Design review of the part shown in the three views and the two pictorial views. Dimensions are in mm from the part's minimum x, y and z. Round coordinates to 2 decimals unless told otherwise and drop trailing zeros. Loops run counter-clockwise (first coordinate to the right, second up) from the corner with the lowest first, then second, coordinate; pieces in that order, holes last. Notation, with made-up numbers: M -29,48.25 L -6,48.25 A30 cw -6,84.25 Z; hole C 61,-22.75 d6. An arc over 180 degrees is marked long. Return JSON: item names as keys, results as strings. Group by question number.
Q1. Consider section D-D (y = 51.5). State the section outline as (x, z) points, and give its area (3 significant figures).
Q2. Consider section A-A (y = 76). State the section outline as (x, z) points.
Q3. Consider section C-C (x = 104). State the section outline as (y, z) points, and give its area (3 significant figures).
Q4. To check wall thickness, follow line 1 along Y through (x, z) = (166.6, 15); line 2 along Z through (x, y) = (166.95, 76); line 3 along X through (y, z) = (67.5, 11). State the ranges of each line that lie inside material, in increasing order.
Q5. Consider section B-B (z = 15). State the section outline as (x, y) points.
Q6. Clearance check with flat-ended pins moving along their axes: pin 1 Ø10 at (x, y) = (59, 39.5) entering from +Z; pin 2 Ø3 at (y, z) = (76, 15) entering from +X; pin 3 Ø2.5 at (x, z) = (166.5, 13) entering from -Y. State where each tip first meets the part, or that it passes through.
Q7. Draft analysis for pull direction X (two halves, no side actions). For the marked faces 1 and 2, state which applies: pulls with the +X half, pulls with the -X half, needs draft (parallel to the pull), parting line crosses it, or undercut.
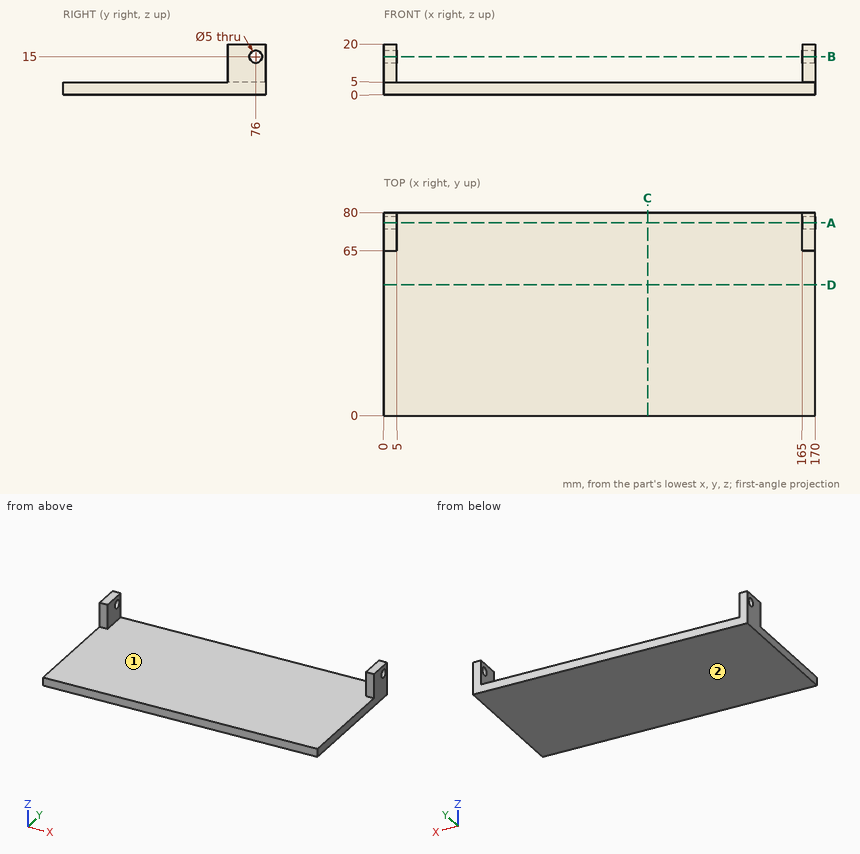
Values:
{
 "1": {"outline": "M 0,0 L 170,0 L 170,5 L 0,5 Z", "area": "850 mm2"},
 "2": {"outline": "M 0,0 L 170,0 L 170,12.5 L 165,12.5 L 165,5 L 5,5 L 5,12.5 L 0,12.5 Z; M 0,17.5 L 5,17.5 L 5,20 L 0,20 Z; M 165,17.5 L 170,17.5 L 170,20 L 165,20 Z"},
 "3": {"outline": "M 0,0 L 80,0 L 80,5 L 0,5 Z", "area": "400 mm2"},
 "4": {"line 1": "y = 65 to 73.5, 78.5 to 80", "line 2": "z = 0 to 12.5, 17.5 to 20", "line 3": "x = 0 to 5, 165 to 170"},
 "5": {"outline": "M 0,65 L 5,65 L 5,73.5 L 0,73.5 Z; M 0,78.5 L 5,78.5 L 5,80 L 0,80 Z; M 165,65 L 170,65 L 170,73.5 L 165,73.5 Z; M 165,78.5 L 170,78.5 L 170,80 L 165,80 Z"},
 "6": {"pin 1": "stops at z = 5", "pin 2": "passes through", "pin 3": "stops at y = 65"},
 "7": {"face 1": "undercut", "face 2": "needs draft"}
}
